Here's the drawing with two shaded views (mm, measured from the low corner). I have some questions. A direction names the side the tool comes from. Coordinates: 2 decimals unless noted, no trailing zeros. Loops run counter-clockwise (first coordinate to the right, second up) from the corner with the lowest first, then second, coordinate; pieces in that order, holes last.
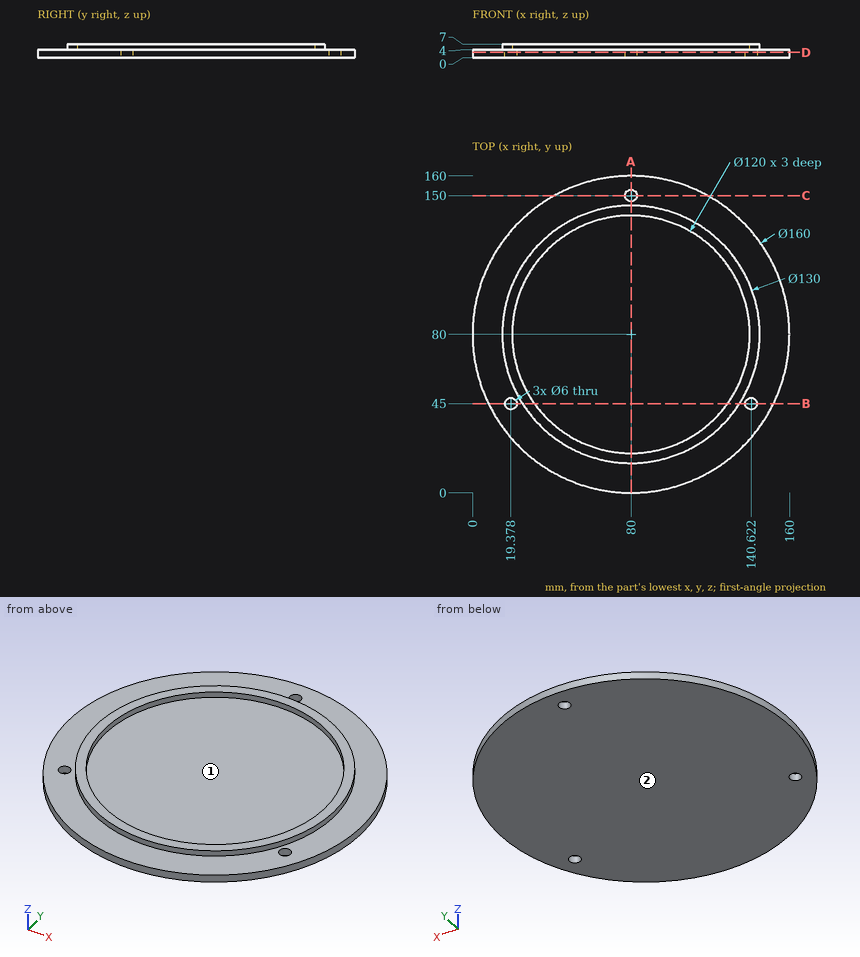
(1) I want a section at A-A on x = 80. Write out the boundary of the cut face in (y, z), then the cut area to 3 significant figures.
Check values:
outline: (0, 0) - (147, 0) - (147, 4) - (145, 4) - (145, 7) - (140, 7) - (140, 4) - (20, 4) - (20, 7) - (15, 7) - (15, 4) - (0, 4) - close; (153, 0) - (160, 0) - (160, 4) - (153, 4) - close
area: 646 mm2
(2) If I drill on probe 1 along Y at (x, z) = (80, 2.4); probe 2 along X at (y, z) = (150, 1.5); probe 3 along Z at (x, y) = (26, 71), over which ranges is the centre line in solid material (lowest first)?
Check values:
probe 1: y = 0 to 147, 153 to 160
probe 2: x = 41.27 to 77, 83 to 118.73
probe 3: z = 0 to 4
(3) I want a section at D-D on z = 2.75. Write out the boundary of the cut face in (x, y).
Check values:
outline: circle Ø160 at (80, 80); hole circle Ø6 at (19.38, 45); hole circle Ø6 at (80, 150); hole circle Ø6 at (140.62, 45)
(4) I'm going to push flat-ended pins straight in: pin 1 (1.5 mm diameter, centred on y = 44.5, z = 5, fed in from -X); pin 2 (1.5 mm diameter, centred on x = 102.5, z = 2, fed in from +Y); pin 3 (6 mm diameter, centred on x = 126.5, y = 79, fed in from +Z). Where does each tip first touch, or does it pass through?
Check values:
pin 1: stops at x = 25.07
pin 2: stops at y = 156.99
pin 3: stops at z = 4
(5) I want a section at C-C on y = 150. Write out the boundary of the cut face in (x, z), then the cut area to 3 significant figures.
Check values:
outline: (41.27, 0) - (77, 0) - (77, 4) - (41.27, 4) - close; (83, 0) - (118.73, 0) - (118.73, 4) - (83, 4) - close
area: 286 mm2
(6) I want a section at B-B on y = 45. Write out the boundary of the cut face in (x, z).
Check values:
outline: (8.06, 0) - (16.38, 0) - (16.38, 4) - (8.06, 4) - close; (22.38, 0) - (137.62, 0) - (137.62, 4) - (134.77, 4) - (134.77, 7) - (128.73, 7) - (128.73, 4) - (31.27, 4) - (31.27, 7) - (25.23, 7) - (25.23, 4) - (22.38, 4) - close; (143.62, 0) - (151.94, 0) - (151.94, 4) - (143.62, 4) - close
(7) Which directions (+Z, -Z, +X, -X, +Y, -Y) give clear straight access to the entire face, cutting with the end or side of a thin tool? Please do the marked faces 1 and 2.
Check values:
face 1: +Z
face 2: -Z, +X, -X, +Y, -Y
